Work out the finished part from the listing and answer in its coordinate system (mm). Face numbers are marked on the shaded views. A direction names the side the tool comes from. Round coordinates to 2 decimals unless told otherwise and drop trailing zeros. Order: outer loops, then holes, each group sorted by start corner. A loop starts at its lowest first (then second) coordinate and runs counter-clockwise, first axis right, second up. Notation, with made-up numbers: (5.25, 34) - (51.25, 34) arc R24 ccw to (51.25, 49) - close; hole circle Ø9 at (-30, 47). An arc over 180 degrees is marked (long way). One line per question, with ' | ' between items. Start each with the question number.
from build123d import *

# Parameters (mm, degrees)
F1_DEPTH = 120
F2_R     = 6
F3_DEPTH = 5


with BuildPart() as f1:
    # F0 (on Top) → F1 (new body)
    with BuildSketch(Plane.XY):
        with BuildLine():
            Line((120.464271, 36.765282), (-39.183099, 36.765282))
            ThreePointArc((-39.183099, 36.765282), (-50.372007, 32.173501), (-54.535729, 20.818346))
            Line((-54.535729, 20.818346), (-54.535729, -83.234718))
            Line((-54.535729, -83.234718), (-49.535177, -83.234718))
            Line((-49.535177, -83.234718), (-49.536819, 10.563834))
            Line((-49.536819, 10.563834), (-49.537028, 22.530258))
            ThreePointArc((-49.537028, 22.530258), (-46.279821, 29.181243), (-39.340395, 31.767623))
            Line((-39.340395, 31.767623), (-28.383342, 31.767623))
            Line((-28.383342, 31.767623), (120.464271, 31.767623))
            Line((120.464271, 31.767623), (120.464271, 36.765282))
        make_face()
    extrude(amount=F1_DEPTH)

    # F2 (on face) → F3 (cut)
    with BuildSketch(Plane(origin=(0, 36.765282, 0), x_dir=(-1, 0, 0), z_dir=(0, 1, 0))):
        with Locations((-70.464271, 60)):
            Circle(F2_R)
        with Locations((-20.464271, 60)):
            Circle(F2_R)
    extrude(amount=-F3_DEPTH, mode=Mode.SUBTRACT)


solid = f1.part
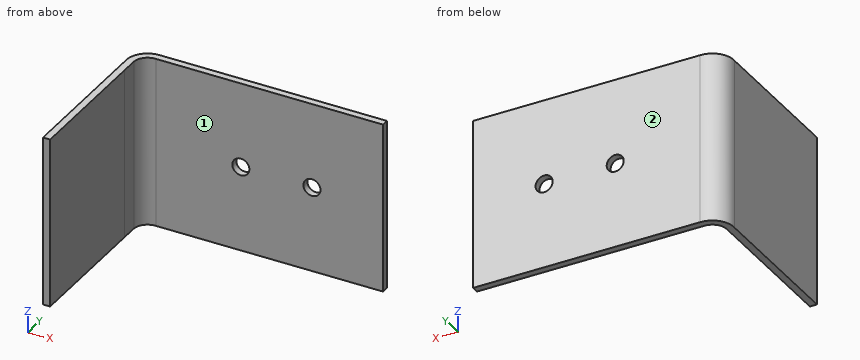
1) Section B-B on z = 92 is taken. Give the vertices of the cut face in (x, y).
2) Flat-ended cylindrical pins translate along their axes: pin 1 (1 mm diameter, centred on x = 72, z = 39.5, fed in from -Y); pin 2 (5 mm diameter, centred on y = 24, z = 48.5, fed in from +X); pin 3 (19 mm diameter, centred on x = 20.46, z = 60, fed in from +Y). Find the tip coordinate at first contact, or state that the pin passes through.
3) Section C-C on x = 107 is taken. Give the vertices of the cut face in (y, z), and give its area (3 significant figures).
4) Section A-A on z = 60 is taken. Give the vertices of the cut face in (x, y), and give its area (3 significant figures).
5) Straight lines are drawn through the part: line 1 (Y direction, x = 113, z = 27); line 2 (X direction, y = -73.5, z = 14); line 3 (X direction, y = 27, z = 14.5). For each, find the intervals that lie inside material, in ascending order.
6) Section D-D on y = -8 is taken. Give the vertices of the cut face in (x, z), and give its area (3 significant figures).
7) For the marked faces 1 and 2, determine the directions among +Z, -Z, +X, -X, +Y, -Y from which every point of the face is accessible in a straight line to the end or side of a thin tool.
Recorded:
1) outline: (-54.54, -83.23) - (-49.54, -83.23) - (-49.54, 22.53) arc R10 cw to (-39.34, 31.77) - (120.46, 31.77) - (120.46, 36.77) - (-39.18, 36.77) arc R15 ccw to (-54.54, 20.82) - close
2) pin 1: stops at y = 31.77 | pin 2: stops at x = -48.38 | pin 3: stops at y = 36.77
3) outline: (31.77, 0) - (36.77, 0) - (36.77, 120) - (31.77, 120) - close | area: 600 mm²
4) outline: (-54.54, -83.23) - (-49.54, -83.23) - (-49.54, 22.53) arc R10 cw to (-39.34, 31.77) - (14.46, 31.77) - (14.46, 36.77) - (-39.18, 36.77) arc R15 ccw to (-54.54, 20.82) - close; (26.46, 31.77) - (64.46, 31.77) - (64.46, 36.77) - (26.46, 36.77) - close; (76.46, 31.77) - (120.46, 31.77) - (120.46, 36.77) - (76.46, 36.77) - close | area: 1,300 mm²
5) line 1: y = 31.77 to 36.77 | line 2: x = -54.54 to -49.54 | line 3: x = -53.62 to -48.09
6) outline: (-54.54, 0) - (-49.54, 0) - (-49.54, 120) - (-54.54, 120) - close | area: 600 mm²
7) face 1: +Z, -Z, +X, -Y | face 2: +Z, -Z, +X, -X, +Y
